For this review, take the finished solid that the model builds, in its own axes (mm). Give positions to 0.01 mm unless a question says otherwise; leave off trailing zeros. Order: outer loops, then holes, each group sorted by start corner. A loop starts at its lowest first (then second) coordinate and runs counter-clockwise, first axis right, second up.
from build123d import *

# Parameters (mm, degrees)
SKETCH_W      = 160
SKETCH_H      = 100
PAD_DEPTH     = 2
CHAMFER_SIZE2 = 4
CHAMFER_SIZE  = 1.5
SKETCH001_R   = 5
POCKET_DEPTH  = 2


with BuildPart() as part:
    # Sketch → Pad (new body)
    with BuildSketch(Plane.XY):
        Rectangle(SKETCH_W, SKETCH_H)
    extrude(amount=PAD_DEPTH)

    # Chamfer
    chamfer_edges = [part.edges().sort_by_distance(p)[0] for p in [
        (0, 50, 2),
    ]]
    chamfer_side = part.faces().sort_by_distance((0, 50, 1))[0]
    chamfer(chamfer_edges, length=CHAMFER_SIZE, length2=CHAMFER_SIZE2, reference=chamfer_side)

    # Sketch001 (on Face5 of Chamfer) → Pocket (cut)
    with BuildSketch(Plane.XY.offset(2)):
        with Locations((-50, -30)):
            Circle(SKETCH001_R)
        with Locations((50, -30)):
            Circle(SKETCH001_R)
    extrude(amount=-POCKET_DEPTH, mode=Mode.SUBTRACT)


solid = part.part
1) Draft analysis for pull direction X (two halves, no side actions). For faces 1 (the face through (-1, 1, 0)), 2 (the face through (46, -33, 1)), 3 (the face through (-54, -33, 1)), state which applies: +X half, -X half, draft (parallel to the pull), parting line (faces both ways), or undercut.
Answer sheet:
face 1: draft
face 2: undercut
face 3: undercut
2) We need section B-B on y = -30. Give the boundary of the cut face in (x, z).
Answer sheet:
outline: (-80, 0) - (-55, 0) - (-55, 2) - (-80, 2) - close; (-45, 0) - (45, 0) - (45, 2) - (-45, 2) - close; (55, 0) - (80, 0) - (80, 2) - (55, 2) - close
3) We need section A-A on x = 50. Give the boundary of the cut face in (y, z), then the cut area to 3 significant figures.
Answer sheet:
outline: (-50, 0) - (-35, 0) - (-35, 2) - (-50, 2) - close; (-25, 0) - (50, 0) - (50, 0.5) - (46, 2) - (-25, 2) - close
area: 177 mm2
4) We need section C-C on z = 0.95. Give the boundary of the cut face in (x, y), then the cut area to 3 significant figures.
Answer sheet:
outline: (-80, -50) - (80, -50) - (80, 48.8) - (-80, 48.8) - close; hole circle Ø10 at (-50, -30); hole circle Ø10 at (50, -30)
area: 15,700 mm2
5) Clearance check with a flat-ended pin moving along its axis: pin 1 (9 mm diameter, centred on x = -50, y = -30, fed in from -Z). State where the tip first meets the part, or that it passes through.
Answer sheet:
pin 1: passes through
6) We need section D-D on x = 11. Give the boundary of the cut face in (y, z), then the cut area to 3 significant figures.
Answer sheet:
outline: (-50, 0) - (50, 0) - (50, 0.5) - (46, 2) - (-50, 2) - close
area: 197 mm2
7) To check wall thickness, follow line 1 (X direction, y = -32, z = 0.3). State the ranges of the line that lie inside material, in increasing order.
Answer sheet:
line 1: x = -80 to -54.58, -45.42 to 45.42, 54.58 to 80
